Can you work these out from the model? Positions are in its coordinate system, mm. Face numbers are marked on the shaded views. A direction names the side the tool comes from. Give positions to 0.01 mm unless a question says otherwise; leave off trailing zeros. Loops run counter-clockwise (first coordinate to the right, second up) from the corner with the lowest first, then second, coordinate; pieces in that order, holes last. Notation, with made-up numbers: (51, 81) - (98, 81) arc R8 ccw to (98, 93) - close; hole circle Ø11 at (-26.75, 49). An arc over 180 degrees is marked (long way). Answer as a JSON object with one key per item and string values.
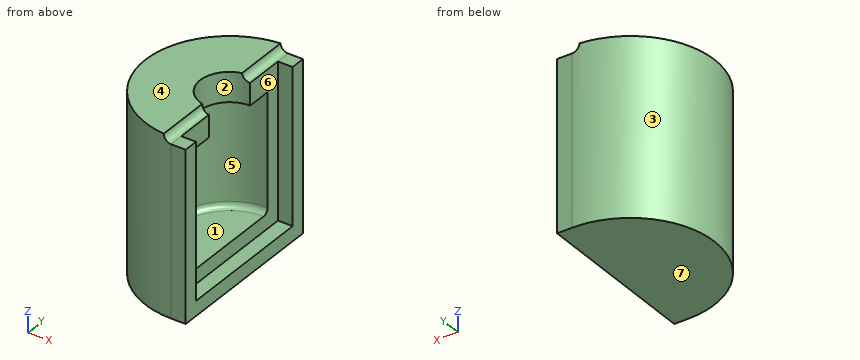
```python
from build123d import *

# Parameters (mm, degrees)
F1_ANGLE_BACK = 90
F1_ANGLE      = 180
F2_R          = 2.5
F3_DEPTH      = 28.501
F3_DEPTH_BACK = 28.501
F4_R          = 1.905
F6_DEPTH      = 5


with BuildPart() as f1:
    # F0 (on Front) → F1 (revolve)
    with BuildSketch(Plane.XZ, mode=Mode.PRIVATE) as f1_sk:
        Polygon((-18.5, 0), (0, 0), (0, 10), (-18.5, 10), (-18.5, 50), (-10, 50), (-10, 60), (-18.5, 60), (-28.5, 60), (-28.5, 0), align=None)
    revolve(f1_sk.sketch.rotate(Axis((0, 0, 5), (0, 0, 1)), -F1_ANGLE_BACK), axis=Axis((0, 0, 5), (0, 0, 1)), revolution_arc=F1_ANGLE)

    # F2 (on Front) → F3 (cut, two sides)
    with BuildSketch(Plane.XZ) as f3_sk:
        with Locations((0, 60)):
            Circle(F2_R)
    extrude(amount=-F3_DEPTH, mode=Mode.SUBTRACT)
    extrude(f3_sk.sketch, amount=F3_DEPTH_BACK, mode=Mode.SUBTRACT)

    # F4
    f4_edges = [f1.edges().sort_by_distance(p)[0] for p in [
        (-18.5, 0, 10),
    ]]
    fillet(f4_edges, radius=F4_R)

    # F5 (on face) → F6 (join)
    with BuildSketch(Plane.YZ):
        Polygon((-23.5, 57.5), (-28.5, 57.5), (-28.5, 0), (28.5, 0), (28.5, 57.5), (23.5, 57.5), (23.5, 54.5), (23.5, 5), (-23.5, 5), (-23.5, 54.5), align=None)
    extrude(amount=F6_DEPTH)


solid = f1.part
```
1) Imagine slicing it at A-A on z = 27.5. Write out the boundary of the cut face in (x, y), and give its area (3 significant figures).
Check sheet entries:
{"outline": "(0, -28.5) - (5, -28.5) - (5, -23.5) - (0, -23.5) - (0, -18.5) arc R18.5 cw to (0, 18.5) - (0, 23.5) - (5, 23.5) - (5, 28.5) - (0, 28.5) arc R28.5 ccw to start", "area": "788 mm2"}
2) I'm going to push flat-ended pins straight in: P1, Ø1, axis at y = 8, z = 41, coming from the +X side; P2, Ø6, axis at x = -20.5, z = 33, coming from the -Y side; P3, Ø10, axis at x = -5.5, z = 50, coming from the -Y side. Where does each tip first touch, or does it pass through?
Check sheet entries:
{"P1": "x = -16.43", "P2": "y = -22.49", "P3": "y = -28.5"}
3) Imagine slicing it at D-D on y = 20. Write out the boundary of the cut face in (x, z), and give its area (3 significant figures).
Check sheet entries:
{"outline": "(-20.3, 0) - (5, 0) - (5, 5) - (0, 5) - (0, 57.5) arc R2.5 cw to (-2.5, 60) - (-20.3, 60) - close", "area": "1,240 mm2"}
4) Imagine slicing it at C-C on x = -26. Write out the boundary of the cut face in (y, z).
Check sheet entries:
{"outline": "(-11.67, 0) - (11.67, 0) - (11.67, 60) - (-11.67, 60) - close"}
5) If we mould it in two halves opening along Z, with no side actions, what happens to the marked faces 4, 5, 6 and 7? For each: released by +Z, released by -Z, zero draft, split by the parting line, or undercut.
Check sheet entries:
{"face 4": "released by +Z", "face 5": "undercut", "face 6": "zero draft", "face 7": "released by -Z"}
6) I need wall thicknesses on L1, parallel to Z at x = -3, y = -7; L2, parallel to Y at x = 1.5, z = 13.5; L3, parallel to Z at x = 3, y = -2.5. Which ranges of each line are inside material? Lowest first, please.
Check sheet entries:
{"L1": "0 to 10", "L2": "-28.5 to -23.5, 23.5 to 28.5", "L3": "0 to 5"}
7) Imagine slicing it at B-B on y = 0. Write out the boundary of the cut face in (x, z) (3 decimals).
Check sheet entries:
{"outline": "(-28.5, 0) - (5, 0) - (5, 5) - (0, 5) - (0, 10) - (-16.595, 10) arc R1.905 cw to (-18.5, 11.905) - (-18.5, 50) - (-10, 50) - (-10, 60) - (-28.5, 60) - close"}
8) Which directions (+Z, -Z, +X, -X, +Y, -Y) give clear straight access to the entire face, cutting with the end or side of a thin tool? Please do the marked faces 1, 2 and 3.
Check sheet entries:
{"face 1": "+X", "face 2": "+Z, +X", "face 3": "+Z, -Z, -X"}
